from build123d import *

# Parameters (mm, degrees)
BOSS_EXTRUDE1_DEPTH = 76.2
FILLET1_R           = 3.175
SKETCH2_R           = 10.414
SKETCH2_R_2         = 1.651
CUT_EXTRUDE2_DEPTH  = 142.990316571
SKETCH4_W           = 68.58
SKETCH4_H           = 76.2
CUT_EXTRUDE3_DEPTH  = 141.599095392
CUT_EXTRUDE4_DEPTH  = 103.644366748


with BuildPart() as part:
    # Sketch1 → Boss-Extrude1 (new body)
    with BuildSketch(Plane.XY):
        Polygon((0, 0), (0, 63.5), (3.175, 63.5), (3.175, 3.175), (101.6, 3.175), (101.6, 0), align=None)
    extrude(amount=BOSS_EXTRUDE1_DEPTH)

    # Fillet1
    fillet1_edges = [part.edges().sort_by_distance(p)[0] for p in [
        (3.175, 3.175, 38.1),
    ]]
    fillet(fillet1_edges, radius=FILLET1_R)

    # Sketch2 → Cut-Extrude2 (cut, through all)
    with BuildSketch(Plane.ZY):
        with Locations((38.1, 38.1)):
            Circle(SKETCH2_R)
        with Locations((38.1, 53.1)):
            Circle(SKETCH2_R_2)
        with Locations((25.109618943, 30.6)):
            Circle(SKETCH2_R_2)
        with Locations((51.090381057, 30.6)):
            Circle(SKETCH2_R_2)
    extrude(amount=-CUT_EXTRUDE2_DEPTH, mode=Mode.SUBTRACT)

    # Sketch4 → Cut-Extrude3 (cut, through all)
    with BuildSketch(Plane(origin=(0, 3.175, 0), x_dir=(1, 0, 0), z_dir=(0, 1, 0))):
        with Locations((67.31, -38.1)):
            Rectangle(SKETCH4_W, SKETCH4_H)
    extrude(amount=-CUT_EXTRUDE3_DEPTH, mode=Mode.SUBTRACT)

    # Sketch5 → Cut-Extrude4 (cut, through all)
    with BuildSketch(Plane(origin=(0, 3.175, 0), x_dir=(1, 0, 0), z_dir=(0, 1, 0))):
        with BuildLine():
            Line((22.86, -12.065), (22.86, -18.415))
            ThreePointArc((22.86, -18.415), (19.685, -21.59), (16.51, -18.415))
            Line((16.51, -18.415), (16.51, -12.065))
            ThreePointArc((16.51, -12.065), (19.685, -8.89), (22.86, -12.065))
        make_face()
        with BuildLine():
            Line((22.86, -64.135), (22.86, -57.785))
            ThreePointArc((22.86, -57.785), (19.685, -54.61), (16.51, -57.785))
            Line((16.51, -57.785), (16.51, -64.135))
            ThreePointArc((16.51, -64.135), (19.685, -67.31), (22.86, -64.135))
        make_face()
    extrude(amount=-CUT_EXTRUDE4_DEPTH, mode=Mode.SUBTRACT)


solid = part.part
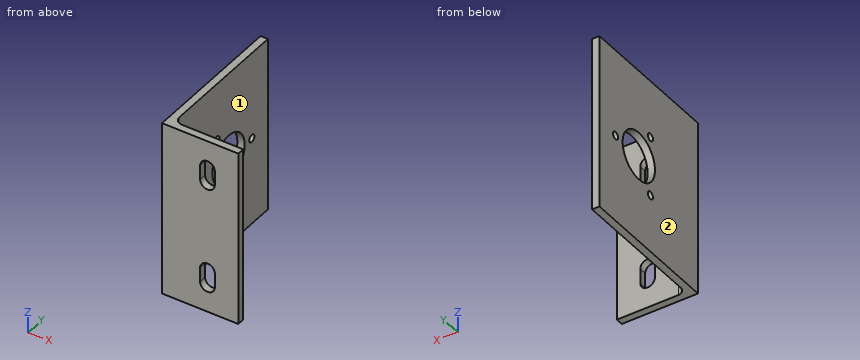
For this review, take the finished solid that the model builds, in its own axes (mm). Face numbers are marked on the shaded views. A direction names the side the tool comes from. Round coordinates to 2 decimals unless told otherwise and drop trailing zeros. Loops run counter-clockwise (first coordinate to the right, second up) from the corner with the lowest first, then second, coordinate; pieces in that order, holes last. Notation, with made-up numbers: (78.5, 77.25) - (108.5, 77.25) arc R17 cw to (108.5, 100.25) - close; hole circle Ø1 at (84.5, -2.5). An arc over 180 degrees is marked (long way). Put each result on its own line as item: value. Start each with the question number.
1. For the marked faces 1 and 2, list the 3-axis set-ups (+Z, -Z, +X, -X, +Y, -Y) from which the entire face can be reached by the end or side of a thin tool; tool diameter is ignored.
2. Consider section C-C on x = 21. State the section outline as (y, z) points (3 decimals).
3. Consider section A-A on z = 38.1. State the section outline as (x, y) points (3 decimals), plus the area to 3 significant figures.
4. Insertion check: P1, Ø1.5, axis at x = 13, z = 33, coming from the +Y side (3 decimals). The pin has a flat end and moves straight along its axis. Give the tip position at first contact, or say it passes through.
5. For probe 1 along Y at (x, z) = (2, 38); probe 2 along X at (y, z) = (53, 34) (3 decimals), list the stretches that pass through material, from the lowest coordinate up. Write a range as [from, to].
6. Consider section B-B on y = 38.1. State the section outline as (x, z) points (3 decimals), plus the area to 3 significant figures.
7. Consider section D-D on z = 63. State the section outline as (x, y) points (3 decimals), plus the area to 3 significant figures.
Result sheet:
1. face 1: +Z, -Z, +X, +Y
1. face 2: +Z, -Z, -X, +Y, -Y
2. outline: (0, 0) - (3.175, 0) - (3.175, 9.175) - (0, 9.175) - close; (0, 21.305) - (3.175, 21.305) - (3.175, 54.895) - (0, 54.895) - close; (0, 67.025) - (3.175, 67.025) - (3.175, 76.2) - (0, 76.2) - close
3. outline: (0, 0) - (33.02, 0) - (33.02, 3.175) - (6.35, 3.175) arc R3.175 cw to (3.175, 6.35) - (3.175, 27.686) - (0, 27.686) - close; (0, 48.514) - (3.175, 48.514) - (3.175, 51.449) - (0, 51.449) - close; (0, 54.751) - (3.175, 54.751) - (3.175, 63.5) - (0, 63.5) - close
3. area: 222 mm^2
4. P1: y = 3.175
5. probe 1: [0, 27.69], [48.51, 51.45], [54.75, 63.5]
5. probe 2: [0, 3.175]
6. outline: (0, 0) - (3.175, 0) - (3.175, 27.686) - (0, 27.686) - close; (0, 48.514) - (3.175, 48.514) - (3.175, 76.2) - (0, 76.2) - close
6. area: 176 mm^2
7. outline: (0, 0) - (16.51, 0) - (16.51, 3.175) - (6.35, 3.175) arc R3.175 cw to (3.175, 6.35) - (3.175, 63.5) - (0, 63.5) - close; (22.86, 0) - (33.02, 0) - (33.02, 3.175) - (22.86, 3.175) - close
7. area: 278 mm^2
